Study the drawing (mm; zero at the part's minimum x, y, z) and answer. A direction names the side the tool comes from. Coordinates: 2 decimals unless noted, no trailing zeros. Loops run counter-clockwise (first coordinate to the right, second up) from the corner with the lowest first, then second, coordinate; pieces in that order, holes last. Notation, with made-up numbers: (33.25, -29.75) - (43.25, -29.75) arc R24 cw to (43.25, 1.25) - close; hole circle Ø11 at (24.25, 87.5). An arc over 180 degrees is marked (long way). Use one line per item in the form item = value.
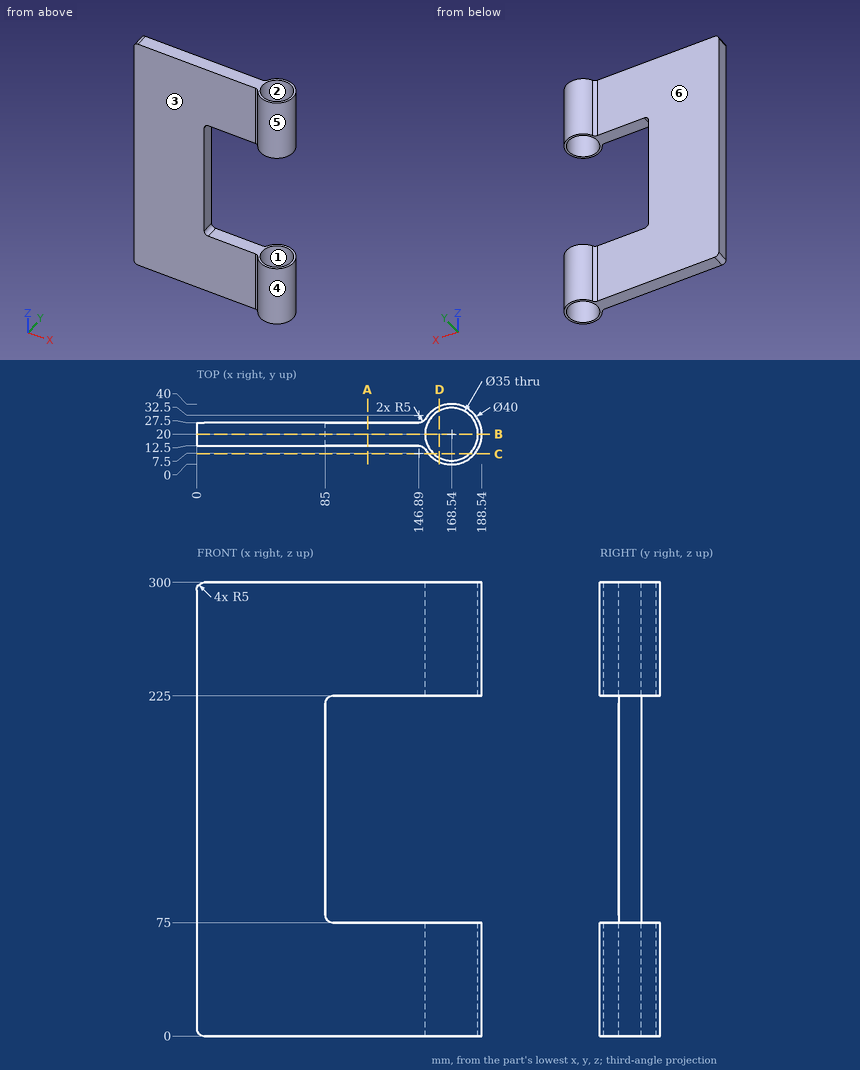
Item 1: Each of these flat-tipped pins is pushed along its axis until it touches: P1, Ø12, axis at x = 164, y = 27.5, coming from the -Z side; P2, Ø12, axis at x = 70, y = 10, coming from the +Z side; P3, Ø1.5, axis at y = 25, z = 74, coming from the +X side; P4, Ø12, axis at y = 18.5, z = 176.5, coming from the +X side. Where does it stop, or does it pass through?
Results below:
P1 = through
P2 = 300
P3 = 188.08
P4 = 85
Item 2: For a pull along X with two mould halves and no side action, classify the marked faces 1, 2, 3 and 4 as +X half, -X half, draft (parallel to the pull), parting line (faces both ways), or undercut.
Results below:
face_1 = undercut
face_2 = undercut
face_3 = draft
face_4 = parting line
Item 3: Which of the six approach directions +Z, -Z, +X, -X, +Y, -Y give full straight-line access (tool end or side, diameter ignored) to the marked faces 5 and 6?
Results below:
face_5 = +Z, -Z
face_6 = +Z, -Z, -X, +Y
Item 4: Find the intervals of material crossed by L1, parallel to Y at x = 49, z = 208; L2, parallel to X at y = 8, z = 46.5 (1 decimal); L3, parallel to Z at x = 115, y = 19.5, in increasing order.
Results below:
L1 = 12.5 to 27.5
L2 = 152.5 to 155.8, 181.3 to 184.5
L3 = 0 to 75, 225 to 300
Item 5: The part is cut by section B-B on y = 20. Give the vertices of the cut face in (x, z).
Results below:
outline = (0, 5) arc R5 ccw to (5, 0) - (151.04, 0) - (151.04, 75) - (90, 75) arc R5 cw to (85, 80) - (85, 220) arc R5 cw to (90, 225) - (151.04, 225) - (151.04, 300) - (5, 300) arc R5 ccw to (0, 295) - close; (186.04, 0) - (188.54, 0) - (188.54, 75) - (186.04, 75) - close; (186.04, 225) - (188.54, 225) - (188.54, 300) - (186.04, 300) - close
Item 6: The part is cut by section A-A on x = 113. Give the vertices of the cut face in (y, z), plus the area to 3 significant figures.
Results below:
outline = (12.5, 0) - (27.5, 0) - (27.5, 75) - (12.5, 75) - close; (12.5, 225) - (27.5, 225) - (27.5, 300) - (12.5, 300) - close
area = 2,250 mm²
Item 7: The part is cut by section C-C on y = 7. Give the vertices of the cut face in (x, z) (1 decimal).
Results below:
outline = (153.3, 0) - (156.8, 0) - (156.8, 75) - (153.3, 75) - close; (153.3, 225) - (156.8, 225) - (156.8, 300) - (153.3, 300) - close; (180.3, 0) - (183.7, 0) - (183.7, 75) - (180.3, 75) - close; (180.3, 225) - (183.7, 225) - (183.7, 300) - (180.3, 300) - close
Item 8: The part is cut by section D-D on x = 160.5. Give the vertices of the cut face in (y, z).
Results below:
outline = (1.69, 0) - (4.46, 0) - (4.46, 75) - (1.69, 75) - close; (1.69, 225) - (4.46, 225) - (4.46, 300) - (1.69, 300) - close; (35.54, 0) - (38.31, 0) - (38.31, 75) - (35.54, 75) - close; (35.54, 225) - (38.31, 225) - (38.31, 300) - (35.54, 300) - close
